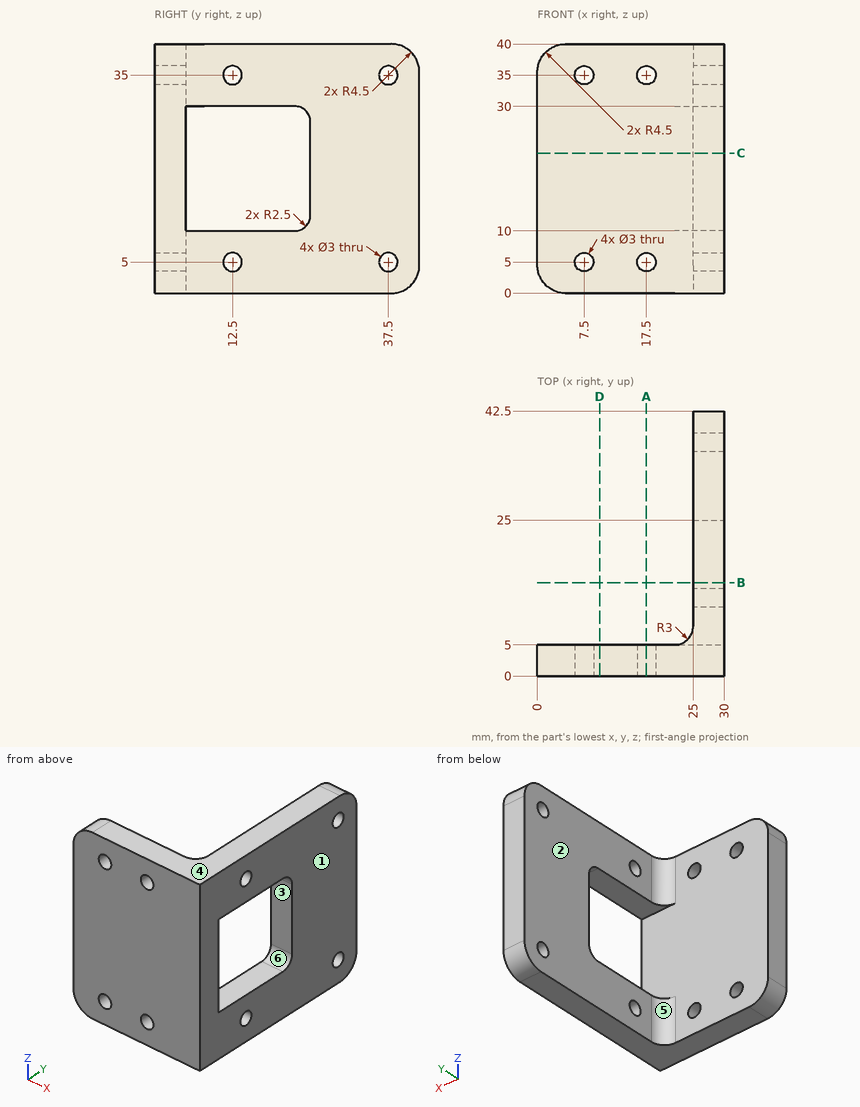
Study the drawing (mm; zero at the part's minimum x, y, z) and answer. A direction names the side the tool comes from. Coordinates: 2 decimals unless noted, no trailing zeros. Write each loop counter-clockwise with the first axis right and the second up, starting at its lowest first coordinate (ties: lowest second). Pieces come first, ordered by that corner, then holes. Notation, with made-up numbers: (25.5, -25.75) - (80.5, -25.75) arc R9 cw to (80.5, -11.75) - close; hole circle Ø1 at (-15, 58). An arc over 180 degrees is marked (long way). Return JSON: item names as keys, results as strings. Group by question number.
1. A cutting plane is placed at D-D, the plane x = 10. Determine the outline of the cut face in (y, z).
2. Straight lines are drawn through the part: L1, parallel to Y at x = 28.8, z = 35; L2, parallel to Z at x = 28, y = 18; L3, parallel to Y at x = 17, z = 37. For each, find the intervals that lie inside material, in ascending order.
3. Given pin 1 (4 mm diameter, centred on x = 7.5, z = 5, fed in from +Y); pin 2 (10.5 mm diameter, centred on y = 22, z = 22, fed in from -X), each flat-ended and moving along its own axis, determine where each tip first touches the part or whether it passes through.
4. A cutting plane is placed at C-C, the plane z = 22.5. Determine the outline of the cut face in (x, y), plus the area to 4 significant figures.
5. Determine the mould class of the marked faces 4, 5 and 6 for opening direction Z: released by +Z, released by -Z, zero draft, split by the parting line, or undercut.
6. Which of the six approach directions +Z, -Z, +X, -X, +Y, -Y give full straight-line access (tool end or side, diameter ignored) to the marked faces 1, 2 and 3?
7. A cutting plane is placed at B-B, the plane y = 15. Determine the outline of the cut face in (x, z).
8. A cutting plane is placed at A-A, the plane x = 17.5. Determine the outline of the cut face in (y, z).
Ans:
{
 "1": {"outline": "(0, 0) - (5, 0) - (5, 40) - (0, 40) - close"},
 "2": {"L1": "0 to 11, 14 to 36, 39 to 42.5", "L2": "0 to 10, 30 to 40", "L3": "0 to 5"},
 "3": {"pin 1": "y = 5", "pin 2": "x = 25"},
 "4": {"outline": "(0, 0) - (30, 0) - (30, 5) - (0, 5) - close; (25, 25) - (30, 25) - (30, 42.5) - (25, 42.5) - close", "area": "237.5 mm²"},
 "5": {"face 4": "released by +Z", "face 5": "zero draft", "face 6": "undercut"},
 "6": {"face 1": "+Z, -Z, +X, +Y, -Y", "face 2": "+Z, -Z, -X, +Y", "face 3": "+X, -X"},
 "7": {"outline": "(25, 0) - (30, 0) - (30, 10) - (25, 10) - close; (25, 30) - (30, 30) - (30, 40) - (25, 40) - close"},
 "8": {"outline": "(0, 0) - (5, 0) - (5, 3.5) - (0, 3.5) - close; (0, 6.5) - (5, 6.5) - (5, 33.5) - (0, 33.5) - close; (0, 36.5) - (5, 36.5) - (5, 40) - (0, 40) - close"}
}
